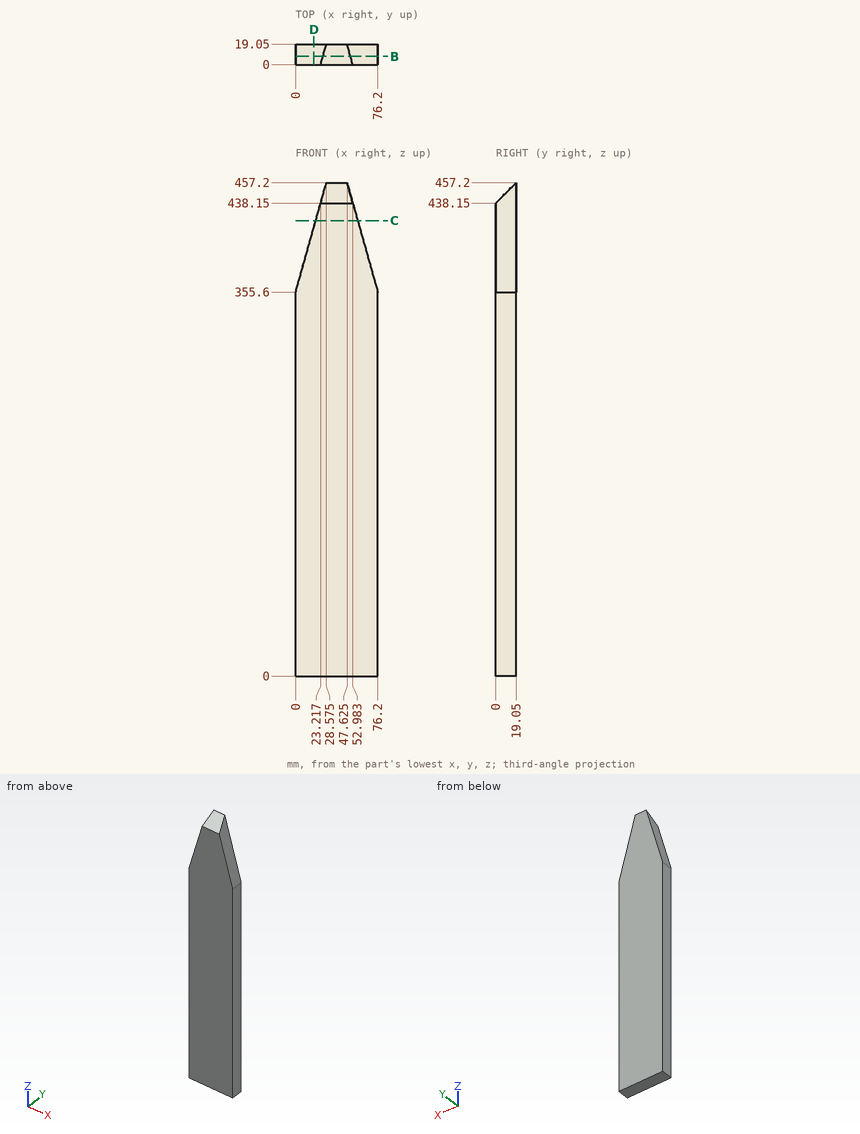
Here's the drawing with two shaded views (mm, measured from the low corner). I have some questions. Give positions to 0.01 mm unless a question says otherwise; leave off trailing zeros. Order: outer loops, then holes, each group sorted by start corner. A loop starts at its lowest first (then second) coordinate and runs counter-clockwise, first axis right, second up.
Q1. If I drill on line 1 along X through (y, z) = (6, 411); line 2 along Z through (x, y) = (48, 11); line 3 along Z through (x, y) = (28.5, 17), over which ranges is the centre line in solid material (lowest first)?
Q2. Suppose I cut it at B-B, the plane y = 7.5. Write out the boundary of the cut face in (x, z), and give its area (3 significant figures).
Q3. Suppose I cut it at C-C, the plane z = 422. Write out the boundary of the cut face in (x, y) (3 decimals), and give its area (3 significant figures).
Q4. Suppose I cut it at D-D, the plane x = 17. Write out the boundary of the cut face in (y, z).
Q5. I'm going to push a flat-ended pin straight in: P1, Ø8, axis at y = 12, z = 355, coming from the -X side. Where does the tip first touch, or does it pass through?
Solution:
1. line 1: x = 15.58 to 60.62
1. line 2: z = 0 to 449.15
1. line 3: z = 0 to 455.15
2. outline: (0, 0) - (76.2, 0) - (76.2, 355.6) - (50.87, 445.65) - (25.33, 445.65) - (0, 355.6) - close
2. area: 31,700 mm2
3. outline: (18.675, 0) - (57.525, 0) - (57.525, 19.05) - (18.675, 19.05) - close
3. area: 740 mm2
4. outline: (0, 0) - (19.05, 0) - (19.05, 416.04) - (0, 416.04) - close
5. P1: stops at x = 0
